For this review, use the dimensioned drawing (mm, ordinates from the lowest corner) and the shaded views. Coordinates: 2 decimals unless noted, no trailing zeros. Loops run counter-clockwise (first coordinate to the right, second up) from the corner with the lowest first, then second, coordinate; pieces in that order, holes last. Notation, with made-up numbers: (-18, 58.5) - (15, 58.5) arc R12 ccw to (15, 69.5) - close; hole circle Ø4 at (10, 78.25). An arc over 180 degrees is marked (long way). Answer in a Markdown table with one row per item. Add a question column.
(1) We need section A-A on x = 17.5. Write out the cut boundary in (y, z), plus the area to 3 significant figures.
(2) We need section D-D on x = 28.5. Write out the cut boundary in (y, z).
(3) For line 1 along X through (y, z) = (2.4, 18); line 2 along Z through (x, y) = (22.5, 1.75); line 3 along Z through (x, y) = (17.5, 1.7), list the stretches that pass through material, from the lowest coordinate up.
(4) For P1, Ø1.5, axis at y = 2.5, z = 10, coming from the -X side; P2, Ø0.9, axis at y = 1, z = 19, coming from the -X side; P3, Ø1.5, axis at x = 1.5, y = 1.5, coming from the +Z side, all flat-tipped, find the tip position at first contact; note any pin that passes through.
(5) We need section B-B on z = 32. Write out the cut boundary in (x, y).
(6) We need section C-C on y = 1.45. Write out the cut boundary in (x, z).
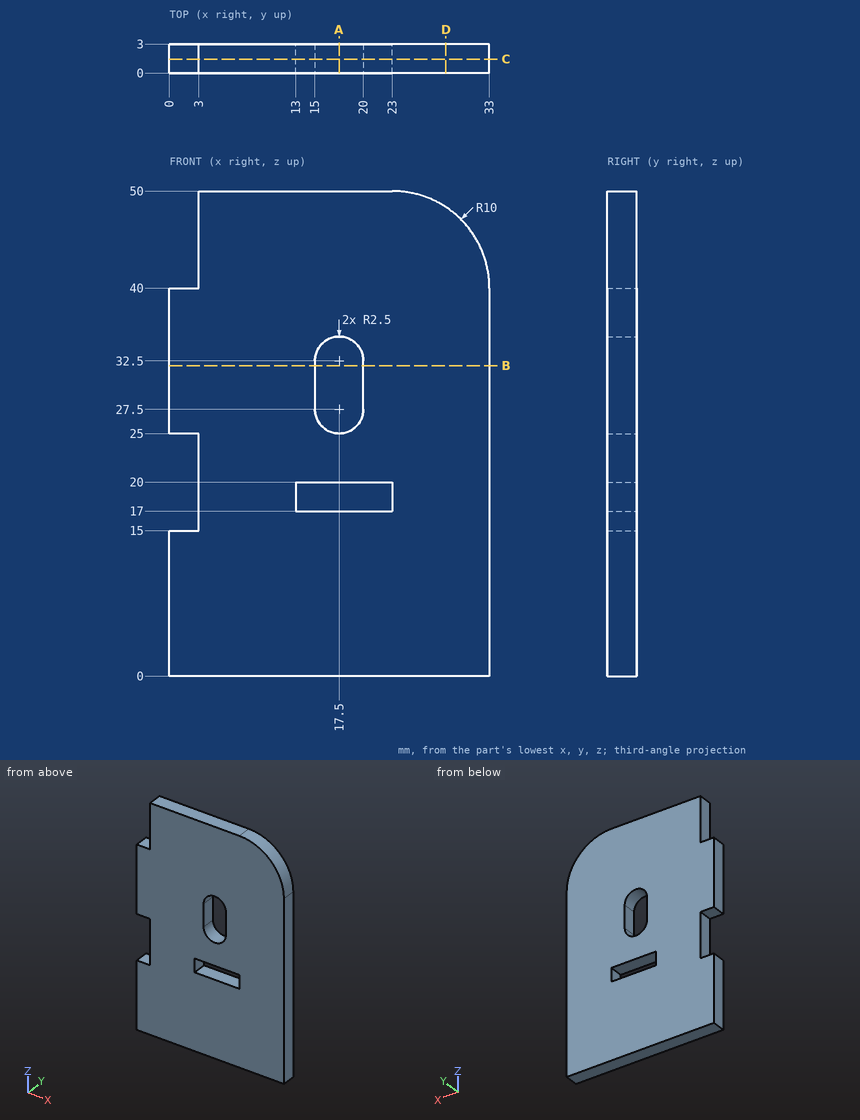
Outcome:
| question | item | result |
|---|---|---|
| 1 | outline | (0, 0) - (3, 0) - (3, 17) - (0, 17) - close; (0, 20) - (3, 20) - (3, 25) - (0, 25) - close; (0, 35) - (3, 35) - (3, 50) - (0, 50) - close |
| 1 | area | 111 mm² |
| 2 | outline | (0, 0) - (3, 0) - (3, 48.35) - (0, 48.35) - close |
| 3 | line 1 | 3 to 13, 23 to 33 |
| 3 | line 2 | 0 to 17, 20 to 50 |
| 3 | line 3 | 0 to 17, 20 to 25, 35 to 50 |
| 4 | P1 | x = 0 |
| 4 | P2 | x = 3 |
| 4 | P3 | z = 40 |
| 5 | outline | (0, 0) - (15, 0) - (15, 3) - (0, 3) - close; (20, 0) - (33, 0) - (33, 3) - (20, 3) - close |
| 6 | outline | (0, 0) - (33, 0) - (33, 40) arc R10 ccw to (23, 50) - (3, 50) - (3, 40) - (0, 40) - (0, 25) - (3, 25) - (3, 15) - (0, 15) - close; hole (13, 17) - (23, 17) - (23, 20) - (13, 20) - close; hole (15, 27.5) arc R2.5 ccw to (20, 27.5) - (20, 32.5) arc R2.5 ccw to (15, 32.5) - close |
